Check sheet for the modelled part. Datum: model origin and axes. Units: mm. Face numbers are marked on the shaded views. A direction names the side the tool comes from. Round coordinates to 2 decimals unless told otherwise and drop trailing zeros. Order: outer loops, then holes, each group sorted by start corner. A loop starts at its lowest first (then second) coordinate and runs counter-clockwise, first axis right, second up. Notation, with made-up numbers: (47, 0) -> (59, 0) arc R14 cw to (59, 25) -> close; hole circle Ø5 at (-23, 18). An arc over 180 degrees is marked (long way). Use CSV: the item, a comma, the result in double quotes.
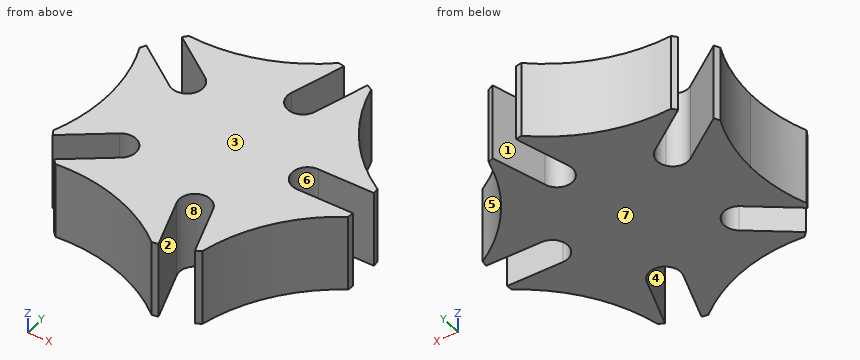
```python
from build123d import *

# Parameters (mm, degrees)
SALIENTE_EXTRUIR1_DEPTH = 5


with BuildPart() as part:
    # Croquis1 → Saliente-Extruir1 (new body)
    with BuildSketch(Plane.XY):
        with BuildLine():
            ThreePointArc((-3.559674775, 2.58625511), (-4.212257305, 2.186352022), (-4.956477022, 2.365023368))
            Line((-4.956477022, 2.365023368), (-7.823412697, 4.447974061))
            ThreePointArc((-7.823412697, 4.447974061), (-7.918450076, 4.276494812), (-8.00972943, 4.102985978))
            ThreePointArc((-8.00972943, 4.102985978), (-7.404365943, 2.091061673), (-7.2, 0))
            ThreePointArc((-7.2, 0), (-7.404365943, -2.091061673), (-8.00972943, -4.102985978))
            ThreePointArc((-8.00972943, -4.102985978), (-7.918450076, -4.276494812), (-7.823412697, -4.447974061))
            Line((-7.823412697, -4.447974061), (-4.956477022, -2.365023368))
            ThreePointArc((-4.956477022, -2.365023368), (-3.559674775, -2.58625511), (-3.780906517, -3.983057357))
            Line((-3.780906517, -3.983057357), (-6.647842193, -6.06600805))
            ThreePointArc((-6.647842193, -6.06600805), (-6.514123901, -6.20938397), (-6.377314065, -6.349812973))
            ThreePointArc((-6.377314065, -6.349812973), (-2.224922359, -6.847606917), (1.427029037, -8.885597763))
            ThreePointArc((1.427029037, -8.885597763), (1.620252616, -8.852403117), (1.812707238, -8.815007201))
            Line((1.812707238, -8.815007201), (0.717635253, -5.444722182))
            ThreePointArc((0.717635253, -5.444722182), (1.359674775, -4.184648672), (2.619748286, -4.826688194))
            Line((2.619748286, -4.826688194), (3.71482027, -8.196973212))
            ThreePointArc((3.71482027, -8.196973212), (3.892500098, -8.114105155), (4.068332581, -8.027386218))
            ThreePointArc((4.068332581, -8.027386218), (5.824922359, -4.232053817), (8.891681878, -1.38861545))
            ThreePointArc((8.891681878, -1.38861545), (8.919821263, -1.194591196), (8.943727382, -1))
            Line((8.943727382, -1), (5.4, -1))
            ThreePointArc((5.4, -1), (4.4, 0), (5.4, 1))
            Line((5.4, 1), (8.943727382, 1))
            ThreePointArc((8.943727382, 1), (8.919821263, 1.194591196), (8.891681878, 1.38861545))
            ThreePointArc((8.891681878, 1.38861545), (5.824922359, 4.232053817), (4.068332581, 8.027386218))
            ThreePointArc((4.068332581, 8.027386218), (3.892500098, 8.114105155), (3.71482027, 8.196973212))
            Line((3.71482027, 8.196973212), (2.619748286, 4.826688194))
            ThreePointArc((2.619748286, 4.826688194), (1.359674775, 4.184648672), (0.717635253, 5.444722182))
            Line((0.717635253, 5.444722182), (1.812707238, 8.815007201))
            ThreePointArc((1.812707238, 8.815007201), (1.620252616, 8.852403117), (1.427029037, 8.885597763))
            ThreePointArc((1.427029037, 8.885597763), (-2.224922359, 6.847606917), (-6.377314065, 6.349812973))
            ThreePointArc((-6.377314065, 6.349812973), (-6.514123901, 6.20938397), (-6.647842193, 6.06600805))
            Line((-6.647842193, 6.06600805), (-3.780906517, 3.983057357))
            ThreePointArc((-3.780906517, 3.983057357), (-3.381003429, 3.330474827), (-3.559674775, 2.58625511))
        make_face()
    extrude(amount=SALIENTE_EXTRUIR1_DEPTH)


solid = part.part
```
Q1. Access from +Z, -Z, +X, -X, +Y, -Y to the whole of each face (thin tool, end or side, straight path). Record for the marked faces 1, 2, 3, 4 and 5.
Result sheet:
face 1,"+Z, -Z, +Y"
face 2,"+Z, -Z"
face 3,"+Z, +X, -X, +Y, -Y"
face 4,"+Z, -Z, -Y"
face 5,"+Z, -Z, +X, +Y"
Q2. Scan lines: L1, parallel to Y at x = -4, z = 1.3; L2, parallel to Y at x = -5, z = 0.4; L3, parallel to X at y = 4.5, z = 0.8. Record each from-to range of solid material in increasing order.
Result sheet:
L1,"y = -6.43 to -4.14, -2.24 to 2.24, 4.14 to 6.43"
L2,"y = -6.33 to -4.87, -2.4 to 2.4, 4.87 to 6.33"
L3,"x = -4.49 to 0.9, 2.44 to 5.64"
Q3. Go/stop test with flat-tipped pins: pin 1 (1.1 mm diameter, centred on x = 7.5, z = 2.5, fed in from +Y); pin 2 (2 mm diameter, centred on y = -6.5, z = 2.5, fed in from +X). Record where each tip stops, or that it passes through.
Result sheet:
pin 1,"stops at y = 2.92"
pin 2,"stops at x = 5.03"
Q4. Sectioned sample at D-D, the plane x = 3. Enter the section's corners in (y, z).
Result sheet:
outline,"(-6, 0) -> (6, 0) -> (6, 5) -> (-6, 5) -> close"
Q5. Sectioned sample at A-A, the plane y = 5.75. Enter the section's corners in (x, z), then the cut area to 3 significant figures.
Result sheet:
outline,"(-6.21, 0) -> (0.82, 0) -> (0.82, 5) -> (-6.21, 5) -> close; (2.92, 0) -> (4.9, 0) -> (4.9, 5) -> (2.92, 5) -> close"
area,"45.1 mm^2"
Q6. Mould release check, pull along X, two halves, no side actions. Record for the marked faces 6, 7 and 8: pulls with the +X half, pulls with the -X half, needs draft (parallel to the pull), parting line crosses it, or undercut.
Result sheet:
face 6,"pulls with the +X half"
face 7,"needs draft"
face 8,"undercut"
Q7. Sectioned sample at C-C, the plane y = -0.5. Enter the section's corners in (x, z).
Result sheet:
outline,"(-7.21, 0) -> (4.53, 0) -> (4.53, 5) -> (-7.21, 5) -> close"
